Verification items for the finished model (mm, model axes). A direction names the side the tool comes from. Coordinates: 2 decimals unless noted, no trailing zeros. Order: outer loops, then holes, each group sorted by start corner. A loop starts at its lowest first (then second) coordinate and runs counter-clockwise, first axis right, second up. Notation, with made-up numbers: M -16,83.25 L 24,83.25 A20 ccw 24,93.25 Z; hole C 47.25,-4 d2. An arc over 180 degrees is marked long. Write item = value, one per line.
```python
from build123d import *

# Parameters (mm, degrees)
PAD003_DEPTH    = 50
SKETCH006_W     = 106.97
SKETCH006_H     = 2
POCKET002_DEPTH = 5
SKETCH007_R     = 2.15
POCKET003_DEPTH = 50.001
FILLET001_R     = 2
SKETCH008_W     = 52.7
SKETCH008_H     = 16.6
POCKET004_DEPTH = 5
SKETCH009_W     = 59
SKETCH009_H     = 9.5
POCKET005_DEPTH = 5


with BuildPart() as part:
    # Sketch005 → Pad003 (new body)
    with BuildSketch(Plane.XY):
        with BuildLine():
            Line((4, 0), (177.97, 0))
            ThreePointArc((181.97, -4), (180.798427, -1.171573), (177.97, 0))
            Line((181.97, -4), (181.97, -101))
            ThreePointArc((177.97, -105), (180.798427, -103.828427), (181.97, -101))
            Line((177.97, -105), (4, -105))
            ThreePointArc((0, -101), (1.171573, -103.828427), (4, -105))
            Line((0, -101), (0, -4))
            ThreePointArc((4, 0), (1.171573, -1.171573), (0, -4))
        make_face()
        with BuildLine():
            Line((10, -3), (171.97, -3))
            ThreePointArc((171.97, -3), (172.434466, -9.535534), (178.97, -10))
            Line((178.97, -10), (178.97, -95))
            ThreePointArc((178.97, -95), (172.434466, -95.464466), (171.97, -102))
            Line((171.97, -102), (10, -102))
            ThreePointArc((10, -102), (9.535534, -95.464466), (3, -95))
            Line((3, -95), (3, -10))
            ThreePointArc((3, -10), (9.535534, -9.535534), (10, -3))
        make_face(mode=Mode.SUBTRACT)
    extrude(amount=PAD003_DEPTH)

    # Sketch006 (on Face17 of Pad003) → Pocket002 (cut)
    with BuildSketch(Plane(origin=(0, 0, 0), x_dir=(1, 0, 0), z_dir=(0, 0, -1))):
        with Locations((113.485, 2)):
            Rectangle(SKETCH006_W, SKETCH006_H)
    extrude(amount=-POCKET002_DEPTH, mode=Mode.SUBTRACT)

    # Sketch007 (on Face4 of Pocket002) → Pocket003 (cut, through all)
    with BuildSketch(Plane(origin=(0, 0, 0), x_dir=(1, 0, 0), z_dir=(0, 0, -1))):
        with Locations((6, 99)):
            Circle(SKETCH007_R)
        with Locations((175.97, 99)):
            Circle(SKETCH007_R)
        with Locations((6, 6)):
            Circle(SKETCH007_R)
        with Locations((175.97, 6)):
            Circle(SKETCH007_R)
    extrude(amount=-POCKET003_DEPTH, mode=Mode.SUBTRACT)

    # Fillet001
    fillet001_edges = [part.edges().sort_by_distance(p)[0] for p in [
        (3, -95, 25),
        (10, -102, 25),
        (3, -10, 25),
        (10, -3, 25),
        (171.97, -102, 25),
        (178.97, -95, 25),
        (178.97, -10, 25),
        (171.97, -3, 25),
    ]]
    fillet(fillet001_edges, radius=FILLET001_R)

    # Sketch008 (on Face24 of Fillet001) → Pocket004 (cut)
    with BuildSketch(Plane.XZ.offset(105)):
        with Locations((38.85, 14.1)):
            Rectangle(SKETCH008_W, SKETCH008_H)
    extrude(amount=-POCKET004_DEPTH, mode=Mode.SUBTRACT)

    # Sketch009 (on Face21 of Pocket004) → Pocket005 (cut)
    with BuildSketch(Plane(origin=(0, 0, 0), x_dir=(0, -1, 0), z_dir=(-1, 0, 0))):
        with Locations((49.5, 8.25)):
            Rectangle(SKETCH009_W, SKETCH009_H)
    extrude(amount=-POCKET005_DEPTH, mode=Mode.SUBTRACT)


solid = part.part
```
Item 1: Sectioned sample at C-C, the plane x = 153. Enter the section's corners in (y, z).
Report:
outline = M -105,0 L -102,0 L -102,50 L -105,50 Z; M -3,5 L -1,5 L -1,0 L 0,0 L 0,50 L -3,50 Z
Item 2: Release check for a two-part mould opening along X. For faces 1 (the flat face through (0, -53, 25)), 2 (the cylindrical face through (9, -10, 25)), 3 (the flat face through (92, -105, 25)) record: pulls with the +X half, pulls with the -X half, needs draft (parallel to the pull), parting line crosses it, or undercut.
Report:
face_1 = pulls with the -X half
face_2 = undercut
face_3 = needs draft
Item 3: Sectioned sample at D-D, the plane y = -72.5. Enter the section's corners in (x, z), then the cut area to 4 significant figures.
Report:
outline = M 0,0 L 3,0 L 3,3.5 L 0,3.5 Z; M 0,13 L 3,13 L 3,50 L 0,50 Z; M 178.97,0 L 181.97,0 L 181.97,50 L 178.97,50 Z
area = 271.5 mm^2
Item 4: Tool access check on faces 4 (the flat face through (3, -53, 25)), 5 (the flat face through (181.97, -52, 25)). Record the directions out of +Z, -Z, +X, -X, +Y, -Y that give a thin tool (end or side, any length) a straight path to the whole face; none if there is none.
Report:
face_4 = +Z, -Z
face_5 = +Z, -Z, +X, +Y, -Y
Item 5: Scan lines: L1, parallel to X at y = -99, z = 32; L2, parallel to Y at x = 6, z = 32; L3, parallel to Y at x = 14, z = 32.5. Record each from-to range of solid material in increasing order. Write a range as from..to.
Report:
L1 = 0..3.85, 8.15..11, 170.97..173.82, 178.12..181.97
L2 = -105..-101.15, -96.85..-94, -11..-8.15, -3.85..0
L3 = -105..-102, -3..0
Item 6: Sectioned sample at A-A, the plane x = 22. Enter the section's corners in (y, z).
Report:
outline = M -105,0 L -102,0 L -102,5.8 L -105,5.8 Z; M -105,22.4 L -102,22.4 L -102,50 L -105,50 Z; M -3,0 L 0,0 L 0,50 L -3,50 Z
Item 7: Sectioned sample at B-B, the plane y = -89.5. Enter the section's corners in (x, z), then the cut area to 3 significant figures.
Report:
outline = M 0,0 L 3,0 L 3,50 L 0,50 Z; M 178.97,0 L 181.97,0 L 181.97,50 L 178.97,50 Z
area = 300 mm^2
Item 8: Gauge pin test, flat ends, axial feed: pin 1 (2.5 mm diameter, centred on x = 1.5, z = 6.5, fed in from -Y); pin 2 (2 mm diameter, centred on y = -2.5, z = 1.5, fed in from -X); pin 3 (2.5 mm diameter, centred on y = -103, z = 13, fed in from -X). Record the tip position at first contact, or that the pin passes through.
Report:
pin_1 = -104.8
pin_2 = 0.03
pin_3 = 0.07
